```python
from build123d import *

# Parameters (mm, degrees)
SKETCH_1_R      = 2.1
EXTRUDE_1_DEPTH = 5
EXTRUDE_START   = 5
SKETCH_1_3_W    = 6
SKETCH_1_3_H    = 12
EXTRUDE_2_DEPTH = 5
FILLET_2_R      = 3


with BuildPart() as part:
    # 草图1 → 凸台-拉伸1 (new body)
    # profile 1 of 2: a face of its own
    with BuildSketch(Plane(origin=(0, 0, 0), x_dir=(1, 0, 0), z_dir=(0, 1, 0))):
        with BuildLine():
            Line((0, 22), (0, 0))
            Line((0, 0), (20, 0))
            Line((20, 0), (20, 22))
            Line((20, 22), (13, 22))
            Line((13, 22), (13, 17.968245837))
            ThreePointArc((13, 17.968245837), (13.862372436, 17.790569415), (14.25, 17))
            ThreePointArc((14.25, 17), (13.862372436, 16.209430585), (13, 16.031754163))
            Line((13, 16.031754163), (13, 10))
            Line((13, 10), (7, 10))
            Line((7, 10), (7, 16.031754163))
            ThreePointArc((7, 16.031754163), (5.75, 17), (7, 17.968245837))
            Line((7, 17.968245837), (7, 22))
            Line((7, 22), (0, 22))
        make_face()
        with Locations(Location((10, 4, 0), (0, 0, 270))):
            Circle(SKETCH_1_R, mode=Mode.SUBTRACT)
    # profile 2 of 2: a face of its own
    with BuildSketch(Plane(origin=(0, 0, 0), x_dir=(1, 0, 0), z_dir=(0, 1, 0))):
        with BuildLine():
            Line((13, 22), (7, 22))
            Line((7, 22), (7, 17.968245837))
            ThreePointArc((7, 17.968245837), (7.540569415, 17.612372436), (7.75, 17))
            ThreePointArc((7.75, 17), (7.540569415, 16.387627564), (7, 16.031754163))
            Line((7, 16.031754163), (7, 10))
            Line((7, 10), (13, 10))
            Line((13, 10), (13, 16.031754163))
            ThreePointArc((13, 16.031754163), (12.25, 17), (13, 17.968245837))
            Line((13, 17.968245837), (13, 22))
        make_face()
    extrude(amount=EXTRUDE_1_DEPTH)

    # 草图1<3> → 凸台-拉伸2 (add)
    with BuildSketch(Plane(origin=(0, 0, 0), x_dir=(1, 0, 0), z_dir=(0, 1, 0)).offset(EXTRUDE_START)):
        with Locations((10, 16)):
            Rectangle(SKETCH_1_3_W, SKETCH_1_3_H)
    extrude(amount=EXTRUDE_2_DEPTH)

    # 圆角2
    fillet_2_edges = [part.edges().sort_by_distance(p)[0] for p in [
        (20, 2.5, 0),
        (0, 2.5, 0),
        (0, 2.5, -22),
        (20, 2.5, -22),
    ]]
    fillet(fillet_2_edges, radius=FILLET_2_R)


solid = part.part
```
Work out the finished part from the listing and answer in its coordinate system (mm). A direction names the side the tool comes from. Give positions to 0.01 mm unless a question says otherwise; leave off trailing zeros. Order: outer loops, then holes, each group sorted by start corner. A loop starts at its lowest first (then second) coordinate and runs counter-clockwise, first axis right, second up. Notation, with made-up numbers: M 18.5,-1 L 71.5,-1 A15 ccw 71.5,4 Z; hole C -38,82 d4. An arc over 180 degrees is marked long. Return JSON: item names as keys, results as strings.
1) Each of these flat-tipped pins is pushed along its axis until it touches: pin 1 (1.5 mm diameter, centred on y = 7, z = -18, fed in from +X); pin 2 (5.5 mm diameter, centred on x = 9, y = 8.5, fed in from +Z); pin 3 (6 mm diameter, centred on x = 9.5, z = -6, fed in from +Y). Where does it stop, or does it pass through?
Resolved:
{"pin 1": "x = 13", "pin 2": "z = -10", "pin 3": "y = 5"}
2) Section D-D, the plane z = -6.5 is taken. Write down the section's boundary in (x, y), plus the area to 3 significant figures.
Resolved:
{"outline": "M 0,0 L 20,0 L 20,5 L 0,5 Z", "area": "100 mm^2"}
3) Section B-B, the plane z = -4 is taken. Write down the section's boundary in (x, y).
Resolved:
{"outline": "M 0,0 L 7.9,0 L 7.9,5 L 0,5 Z; M 12.1,0 L 20,0 L 20,5 L 12.1,5 Z"}
4) For a pull along X with two mould halves and no side action, classify faces 1 (the flat face through (10, 7, -10)), 2 (the flat face through (20, 2, -11)), 3 (the cylindrical face through (12.082, 2.465, -4.273)) as +X half, -X half, draft (parallel to the pull), parting line (faces both ways), or undercut.
Resolved:
{"face 1": "draft", "face 2": "+X half", "face 3": "undercut"}
5) Section C-C, the plane y = 1.5 is taken. Write down the section's boundary in (x, z).
Resolved:
{"outline": "M 0,-19 A3 ccw 3,-22 L 17,-22 A3 ccw 20,-19 L 20,-3 A3 ccw 17,0 L 3,0 A3 ccw 0,-3 Z; hole C 6.75,-17 d2; hole C 10,-4 d4.2; hole C 13.25,-17 d2"}
6) A tool of negligible diameter and unlimited length cuts with its end or side. For faces 4 (the flat face through (7, 7, -16)), 5 (the flat face through (10, 0, -11)), 6 (the flat face through (13, 7, -16)), from which of +Z, -Z, +X, -X, +Y, -Y can it reach the whole face along a straight path? Write none if from no direction.
Resolved:
{"face 4": "+Z, -Z, -X, +Y", "face 5": "+Z, -Z, +X, -X, -Y", "face 6": "+Z, -Z, +X, +Y"}
7) Section A-A, the plane x = 10 is taken. Write down the section's boundary in (y, z), plus the area to 3 significant figures.
Resolved:
{"outline": "M 0,-22 L 10,-22 L 10,-10 L 5,-10 L 5,-6.1 L 0,-6.1 Z; M 0,-1.9 L 5,-1.9 L 5,0 L 0,0 Z", "area": "149 mm^2"}
8) Straight lines are drawn through the part: line 1 along Z through (x, y) = (6.75, 2.5); line 2 along X through (y, z) = (3.5, -17.25); line 3 along X through (y, z) = (3.85, -4). For each, find the intervals that lie inside material, in ascending order. Write a range as [from, to].
Resolved:
{"line 1": "[-22, -18], [-16, 0]", "line 2": "[0, 5.78], [7.72, 12.28], [14.22, 20]", "line 3": "[0, 7.9], [12.1, 20]"}
